from build123d import *

# Parameters (mm, degrees)
SKETCH1_W           = 202
SKETCH1_H           = 72
BOSS_EXTRUDE1_DEPTH = 1.4
SKETCH2_W           = 199
SKETCH2_H           = 69
SKETCH2_W_2         = 197
SKETCH2_H_2         = 67
BOSS_EXTRUDE2_DEPTH = 9
FILLET1_R           = 3.5
FILLET2_R           = 4.5
FILLET3_R           = 6
FILLET4_R           = 3


with BuildPart() as part:
    # Sketch1 → Boss-Extrude1 (new body)
    with BuildSketch(Plane.XY):
        with Locations((101, 36)):
            Rectangle(SKETCH1_W, SKETCH1_H)
    extrude(amount=BOSS_EXTRUDE1_DEPTH)

    # Sketch2 → Boss-Extrude2 (add)
    with BuildSketch(Plane.XY.offset(1.4)):
        with Locations((101, 36)):
            Rectangle(SKETCH2_W, SKETCH2_H)
        with Locations((101, 36)):
            Rectangle(SKETCH2_W_2, SKETCH2_H_2, mode=Mode.SUBTRACT)
    extrude(amount=BOSS_EXTRUDE2_DEPTH)

    # Fillet1
    fillet1_edges = [part.edges().sort_by_distance(p)[0] for p in [
        (2.5, 2.5, 5.9),
        (199.5, 2.5, 5.9),
        (199.5, 69.5, 5.9),
        (2.5, 69.5, 5.9),
    ]]
    fillet(fillet1_edges, radius=FILLET1_R)

    # Fillet2
    fillet2_edges = [part.edges().sort_by_distance(p)[0] for p in [
        (1.5, 70.5, 5.9),
        (1.5, 1.5, 5.9),
        (200.5, 1.5, 5.9),
        (200.5, 70.5, 5.9),
    ]]
    fillet(fillet2_edges, radius=FILLET2_R)

    # Fillet3
    fillet3_edges = [part.edges().sort_by_distance(p)[0] for p in [
        (0, 72, 0.7),
        (202, 72, 0.7),
        (202, 0, 0.7),
        (0, 0, 0.7),
    ]]
    fillet(fillet3_edges, radius=FILLET3_R)

    # Fillet4
    fillet4_edges = [part.edges().sort_by_distance(p)[0] for p in [
        (101, 69.5, 1.4),
        (2.5, 36, 1.4),
        (101, 2.5, 1.4),
        (199.5, 36, 1.4),
        (198.474873734, 3.525126266, 1.4),
        (198.474873734, 68.474873734, 1.4),
        (3.525126266, 3.525126266, 1.4),
        (3.525126266, 68.474873734, 1.4),
    ]]
    fillet(fillet4_edges, radius=FILLET4_R)


solid = part.part
For this review, take the finished solid that the model builds, in its own axes (mm). A direction names the side the tool comes from. Round coordinates to 2 decimals unless told otherwise and drop trailing zeros. Loops run counter-clockwise (first coordinate to the right, second up) from the corner with the lowest first, then second, coordinate; pieces in that order, holes last. Notation, with made-up numbers: (-13, -28) - (17, -28) arc R29 ccw to (17, -2) - close; hole circle Ø8 at (37.25, -31.75). An arc over 180 degrees is marked (long way). One line per item, written item: value. Start each with the question number.
Item 1: For faces 5 (the cylindrical face through (2.783, 2.853, 5.963)), 6 (the flat face through (199.5, 36, 7)), 7 (the cylindrical face through (199.147, 69.217, 5.963)), 8 (the cylindrical face through (199.147, 2.783, 5.963)), list the 3-axis set-ups (+Z, -Z, +X, -X, +Y, -Y) from which the entire face can be reached by the end or side of a thin tool; tool diameter is ignored.
Item 2: Take a section at C-C (y = 32). Give the boundary of the cut face in (x, z).
Item 3: Clearance check with flat-ended pins moving along their axes: pin 1 Ø2 at (y, z) = (22, 7) entering from -X; pin 2 Ø4.5 at (x, z) = (71, 7) entering from -Y; pin 3 Ø12 at (x, y) = (106.5, 57.5) entering from +Z. State where each tip first meets the part, or that it passes through.
Item 4: For L1, parallel to Y at x = 185, z = 4.25; L2, parallel to X at y = 17, z = 9; L3, parallel to Z at x = 63.5, y = 37.5, list the stretches that pass through material, from the lowest coordinate up.
Item 5: Take a section at B-B (x = 183.5). Give the boundary of the cut face in (y, z).
Item 6: The part is to be moulded in two halves that separate along Y. For faces 1 (the cylindrical face through (200.196, 1.711, 0.71)), 2 (the flat face through (1.5, 36, 6)), 3 (the cylindrical face through (2.783, 69.147, 5.963)), 4 (the flat face through (100, 2.5, 7)), say which applies: +Y half, -Y half, draft (parallel to the pull), parting line (faces both ways), or undercut.
Item 7: Take a section at A-A (z = 7.75). Give the boundary of the cut face in (x, y), plus the area to 3 significant figures.
Answer below:
1. face 5: +Z, -X, -Y
1. face 6: +Z
1. face 7: +Z, +X, +Y
1. face 8: +Z, +X, -Y
2. outline: (0, 0) - (202, 0) - (202, 1.4) - (200.5, 1.4) - (200.5, 10.4) - (199.5, 10.4) - (199.5, 4.4) arc R3 cw to (196.5, 1.4) - (5.5, 1.4) arc R3 cw to (2.5, 4.4) - (2.5, 10.4) - (1.5, 10.4) - (1.5, 1.4) - (0, 1.4) - close
3. pin 1: stops at x = 1.5
3. pin 2: stops at y = 1.5
3. pin 3: stops at z = 1.4
4. L1: y = 1.5 to 2.5, 69.5 to 70.5
4. L2: x = 1.5 to 2.5, 199.5 to 200.5
4. L3: z = 0 to 1.4
5. outline: (0, 0) - (72, 0) - (72, 1.4) - (70.5, 1.4) - (70.5, 10.4) - (69.5, 10.4) - (69.5, 4.4) arc R3 cw to (66.5, 1.4) - (5.5, 1.4) arc R3 cw to (2.5, 4.4) - (2.5, 10.4) - (1.5, 10.4) - (1.5, 1.4) - (0, 1.4) - close
6. face 1: -Y half
6. face 2: draft
6. face 3: +Y half
6. face 4: undercut
7. outline: (1.5, 6) arc R4.5 ccw to (6, 1.5) - (196, 1.5) arc R4.5 ccw to (200.5, 6) - (200.5, 66) arc R4.5 ccw to (196, 70.5) - (6, 70.5) arc R4.5 ccw to (1.5, 66) - close; hole (2.5, 6) arc R3.5 ccw to (6, 2.5) - (196, 2.5) arc R3.5 ccw to (199.5, 6) - (199.5, 66) arc R3.5 ccw to (196, 69.5) - (6, 69.5) arc R3.5 ccw to (2.5, 66) - close
7. area: 525 mm2
